Part model, mm, in its own coordinate system. A direction names the side the tool comes from. Give positions to 0.01 mm unless a question says otherwise; leave off trailing zeros. Order: outer loops, then holes, each group sorted by start corner. A loop starts at its lowest first (then second) coordinate and runs counter-clockwise, first axis right, second up.
from build123d import *

# Parameters (mm, degrees)
BOSS_EXTRUDE1_DEPTH     = 45
SKETCH1_3_R             = 6
BOSS_EXTRUDE2_DEPTH     = 10
BOSS_EXTRUDE3_DEPTH     = 35
FILLET1_R               = 12
FILLET2_R               = 12
FILLET3_R               = 12
CUT_EXTRUDE1_DEPTH      = 128.869924602
CUT_EXTRUDE1_DEPTH_BACK = 128.869924602
SKETCH2_R               = 6


with BuildPart() as part:
    # Sketch1 → Boss-Extrude1 (new body)
    with BuildSketch(Plane.XY):
        Polygon((42, 10.408163265), (0, 10.408163265), (0, 0), (30, 0), (30, 4.387755102), (54, 4.387755102), (54, 10.408163265), align=None)
        Polygon((66, 10.408163265), (54, 10.408163265), (54, 4.387755102), (78, 4.387755102), (78, 0), (108, 0), (108, 10.408163265), align=None)
    extrude(amount=BOSS_EXTRUDE1_DEPTH)

    # Sketch1_3 → Boss-Extrude2 (add)
    # profile 1 of 2: a face of its own
    with BuildSketch(Plane.XY):
        Polygon((0, 62), (0, 10.408163265), (42, 10.408163265), (34, 50.265306122), (29, 50.265306122), (29, 62), align=None)
        with Locations((12, 50)):
            Circle(SKETCH1_3_R, mode=Mode.SUBTRACT)
    # profile 2 of 2: a face of its own
    with BuildSketch(Plane.XY):
        Polygon((74, 51.795918367), (66, 10.408163265), (108, 10.408163265), (108, 62), (79, 62), (79, 51.795918367), align=None)
        with Locations((96, 50)):
            Circle(SKETCH1_3_R, mode=Mode.SUBTRACT)
    extrude(amount=BOSS_EXTRUDE2_DEPTH)

    # Sketch1_4 → Boss-Extrude3 (add)
    with BuildSketch(Plane.XY):
        with BuildLine():
            Line((34, 50.265306122), (42, 10.408163265))
            Line((42, 10.408163265), (54, 10.408163265))
            Line((54, 10.408163265), (54, 47))
            ThreePointArc((54, 47), (43.393398282, 51.393398282), (39, 62))
            Line((39, 62), (29, 62))
            Line((29, 62), (29, 50.265306122))
            Line((29, 50.265306122), (34, 50.265306122))
        make_face()
        with BuildLine():
            Line((54, 47), (54, 10.408163265))
            Line((54, 10.408163265), (66, 10.408163265))
            Line((66, 10.408163265), (74, 51.795918367))
            Line((74, 51.795918367), (79, 51.795918367))
            Line((79, 51.795918367), (79, 62))
            Line((79, 62), (69, 62))
            ThreePointArc((69, 62), (64.606601718, 51.393398282), (54, 47))
        make_face()
    extrude(amount=BOSS_EXTRUDE3_DEPTH)

    # Fillet1
    fillet1_edges = [part.edges().sort_by_distance(p)[0] for p in [
        (0, 62, 5),
    ]]
    fillet(fillet1_edges, radius=FILLET1_R)

    # Fillet2
    fillet2_edges = [part.edges().sort_by_distance(p)[0] for p in [
        (108, 62, 5),
    ]]
    fillet(fillet2_edges, radius=FILLET2_R)

    # Fillet3
    fillet3_edges = [part.edges().sort_by_distance(p)[0] for p in [
        (108, 5.204081633, 45),
        (0, 5.204081633, 45),
    ]]
    fillet(fillet3_edges, radius=FILLET3_R)

    # Sketch2 → Cut-Extrude1 (cut, two sides: drawn at the far end of the back side and taken through both)
    with BuildSketch(Plane(origin=(0, 10.408163265, 0), x_dir=(1, 0, 0), z_dir=(0, 1, 0)).offset(-CUT_EXTRUDE1_DEPTH_BACK)):
        with Locations(Location((12, -33, 0), (0, 0, 270))):
            Circle(SKETCH2_R)
        with Locations(Location((96, -33, 0), (0, 0, 270))):
            Circle(SKETCH2_R)
    extrude(amount=CUT_EXTRUDE1_DEPTH + CUT_EXTRUDE1_DEPTH_BACK, mode=Mode.SUBTRACT)


solid = part.part
Item 1: Band-saw the part on A-A on z = 8. List the corners of the cut face in (x, y), plus the area to 3 significant figures.
Item 2: Which spindle directions (+Z, -Z, +X, -X, +Y, -Y) get a long thin tool onto all of the face, cutting with end or side? Do faces 1 (the face through (37.944, 30.616, 22.325)), 2 (the face through (54, 37, 35)), 3 (the face through (54, 4.388, 22)). Say none if no direction does.
Item 3: Band-saw the part on D-D on y = 29. List the corners of the cut face in (x, z), plus the area to 3 significant figures.
Item 4: Pull direction Y, two halves, no side cores. Call faces 4 (the face through (76, 51.796, 22)), 5 (the face through (15, 0, 22)), 6 (the face through (79, 57, 22)): released by +Y, released by -Y, zero draft, split by the parting line, or undercut.
Item 5: Band-saw the part on C-C on x = 52. List the corners of the cut face in (y, z).
Item 6: Drill centre lines: probe 1 along X at (y, z) = (7.5, 32.5); probe 2 along Y at (x, z) = (96, 6); probe 3 along X at (y, z) = (2.5, 33). Where is each one in solid material? Low to high.
Item 7: Band-saw the part on B-B on z = 36.5. List the corners of the cut face in (x, y), plus the area to 3 significant figures.
Item 8: Drop flat-ended pins along their axis: P1, Ø2.5, axis at x = 75.5, z = 21, coming from the -Y side; P2, Ø4, axis at y = 34.5, z = 34.5, coming from the -X side; P3, Ø15, axis at x = 50, y = 38.5, coming from the +Z side; P4, Ø7, axis at x = 12, y = 50, coming from the -Z side. Give the stop position or say it passes through.
Working result:
1. outline: (0, 0) - (30, 0) - (30, 4.39) - (78, 4.39) - (78, 0) - (108, 0) - (108, 50) arc R12 ccw to (96, 62) - (69, 62) arc R15 cw to (39, 62) - (12, 62) arc R12 ccw to (0, 50) - close; hole circle Ø12 at (12, 50); hole circle Ø12 at (96, 50)
1. area: 5,840 mm2
2. face 1: +Z, -X
2. face 2: +Z, +X, -X, +Y
2. face 3: +Z, -Z, -Y
3. outline: (0, 0) - (108, 0) - (108, 10) - (69.59, 10) - (69.59, 35) - (38.27, 35) - (38.27, 10) - (0, 10) - close
3. area: 1,860 mm2
4. face 4: undercut
4. face 5: released by -Y
4. face 6: zero draft
5. outline: (4.39, 0) - (47.13, 0) - (47.13, 35) - (10.41, 35) - (10.41, 45) - (4.39, 45) - close
6. probe 1: x = 0 to 6.02, 17.98 to 90.02, 101.98 to 108
6. probe 2: y = 0 to 44, 56 to 62
6. probe 3: x = 0 to 6, 18 to 30, 78 to 90, 102 to 108
7. outline: (0.52, 0) - (7.13, 0) - (7.13, 10.41) - (0.52, 10.41) - close; (16.87, 0) - (30, 0) - (30, 4.39) - (78, 4.39) - (78, 0) - (91.13, 0) - (91.13, 10.41) - (16.87, 10.41) - close; (100.87, 0) - (107.48, 0) - (107.48, 10.41) - (100.87, 10.41) - close
7. area: 700 mm2
8. P1: stops at y = 4.39
8. P2: stops at x = 36.76
8. P3: stops at z = 35
8. P4: passes through
